```python
from build123d import *

# Parameters (mm, degrees)
BOSS_EXTRUDE1_DEPTH   = 3
SKETCH3_R             = 12.7
BOSS_EXTRUDE2_DEPTH   = 3
F_8_CLEARANCE_HOLE1_D = 4.3053


with BuildPart() as part:
    # Sketch2 → Boss-Extrude1 (new body)
    with BuildSketch(Plane(origin=(0, 0, 0), x_dir=(1, 0, 0), z_dir=(0, 1, 0))):
        with BuildLine():
            Line((-37.697043062, 4.281020581), (-37.697043062, -8.418979419))
            add(Edge.make_bspline(
                [(-37.697043062, -8.418979419), (17.380898097, -15.277400847), (29.368687451, 31.123681561)],
                knots=[0, 0, 0, 1, 1, 1], degree=2))
            Line((29.368687451, 31.123681561), (14.247453118, 35.062826639))
            add(Edge.make_bspline(
                [(-37.697043062, 4.281020581), (6.487978336, -0.323288205), (14.247453118, 35.062826639)],
                knots=[0, 0, 0, 1, 1, 1], degree=2))
        make_face()
    extrude(amount=BOSS_EXTRUDE1_DEPTH)

    # Sketch3 → Boss-Extrude2 (add)
    with BuildSketch(Plane(origin=(0, 0, 0), x_dir=(1, 0, 0), z_dir=(0, 1, 0))):
        with Locations((23.06337647, 37.912010101)):
            Circle(SKETCH3_R)
    extrude(amount=BOSS_EXTRUDE2_DEPTH)

    # #8 Clearance Hole1 (through all)
    with Locations(Plane(origin=(0, 3, 0), x_dir=(1, 0, 0), z_dir=(0, 1, 0))):
        with Locations((-30.855203609, -2.496063835)):
            Hole(F_8_CLEARANCE_HOLE1_D / 2)


solid = part.part
```
Design review of the part built by this model. Coordinates are the model's own, in mm. Coordinates: 2 decimals unless noted, no trailing zeros. Write each loop counter-clockwise with the first axis right and the second up, starting at its lowest first coordinate (ties: lowest second). Pieces come first, ordered by that corner, then holes.
1) To check wall thickness, follow L1, parallel to X at y = 0.55, z = 4; L2, parallel to Z at x = -32.5, y = 2.55; L3, parallel to X at y = 1.8, z = -29. State the ranges of each line that lie inside material, in increasing order.
2) Mouldability with a two-part tool opening along Z and no side actions: class faces 1 (the flat face through (7, 0, -16)), 2 (the cylindrical face through (-28.705, 1.479, 2.401)) as +Z half, -Z half, draft (parallel to the pull), parting line (faces both ways), or undercut.
3) Add section A-A (z = -32). Write out the cut boundary in (x, y), plus the area to 3 significant figures.
Check result:
1. L1: x = -37.7 to -32.4, -29.32 to 2.74
1. L2: z = -3.87 to 1.11, 3.88 to 8.96
1. L3: x = 12.55 to 32.11
2. face 1: draft
2. face 2: undercut
3. outline: (11.82, 0) - (34.3, 0) - (34.3, 3) - (11.82, 3) - close
3. area: 67.4 mm2
